```python
from build123d import *

# Parameters (mm, degrees)
SKETCH1_W           = 12.710924787
SKETCH1_H           = 15.963552005
SKETCH1_R           = 1.8
BOSS_EXTRUDE1_DEPTH = 1
SKETCH2_R           = 1.75
BOSS_EXTRUDE2_DEPTH = 5
SKETCH3_R           = 3.5
BOSS_EXTRUDE3_DEPTH = 5
CHAMFER1_SIZE       = 2


with BuildPart() as part:
    # Sketch1 → Boss-Extrude1 (new body)
    with BuildSketch(Plane.XY.offset(46.41148)):
        with Locations((39.508303211, 7.326783953)):
            Rectangle(SKETCH1_W, SKETCH1_H)
        with Locations((38.478852397, 6.566573863)):
            Circle(SKETCH1_R, mode=Mode.SUBTRACT)
    extrude(amount=BOSS_EXTRUDE1_DEPTH)

    # Sketch2 → Boss-Extrude2 (add)
    with BuildSketch(Plane(origin=(30.5, 0, 0), x_dir=(0, 0, -1), z_dir=(1, 0, 0))):
        with BuildLine():
            Line((-56.841529107, 37.437587441), (-49.41148, 37.437587441))
            Line((-49.41148, 37.437587441), (-49.41148, 17.308559955))
            Line((-49.41148, 17.308559955), (-47.41148, 15.308559955))
            Line((-47.41148, 15.308559955), (-47.41148, 12.308559955))
            Line((-47.41148, 12.308559955), (-52.41148, 12.308559955))
            Line((-52.41148, 12.308559955), (-61.318087937, 30.210387171))
            ThreePointArc((-61.318087937, 30.210387171), (-61.092176196, 35.07045647), (-56.841529107, 37.437587441))
        make_face()
        with Locations((-56.841529107, 32.437587441)):
            Circle(SKETCH2_R, mode=Mode.SUBTRACT)
    extrude(amount=BOSS_EXTRUDE2_DEPTH)

    # Sketch3 → Boss-Extrude3 (add)
    with BuildSketch(Plane.XY.offset(47.41148)):
        Polygon((35.5, 15.308559955), (35.5, 12.308559955), (33.152840817, 12.308559955), (33.152840817, -0.65499205), (45.863765604, -0.65499205), (45.863765604, 15.308559955), align=None)
        with Locations((38.478852397, 6.566573863)):
            Circle(SKETCH3_R, mode=Mode.SUBTRACT)
    extrude(amount=BOSS_EXTRUDE3_DEPTH)

    # Chamfer1
    chamfer1_edges = [part.edges().sort_by_distance(p)[0] for p in [
        (33.152840817, 12.308559955, 49.91148),
    ]]
    chamfer(chamfer1_edges, length=CHAMFER1_SIZE)


solid = part.part
```
Geometry check sheet. Reference: the model listing, model coordinates, mm. A direction names the side the tool comes from. Coordinates: 2 decimals unless noted, no trailing zeros. Order: outer loops, then holes, each group sorted by start corner. A loop starts at its lowest first (then second) coordinate and runs counter-clockwise, first axis right, second up.
Q1. Sectioned sample at A-A on z = 57.5. Record the cut outline in (x, y).
Reply:
outline: (30.5, 22.54) - (35.5, 22.54) - (35.5, 30.82) - (30.5, 30.82) - close; (30.5, 34.06) - (35.5, 34.06) - (35.5, 37.39) - (30.5, 37.39) - close
Q2. Thickness scan on probe 1 along X at (y, z) = (26, 51.5); probe 2 along Z at (x, y) = (42.5, 7); probe 3 along Y at (x, z) = (33, 56.75). Record the ranges inside material, lowest first.
Reply:
probe 1: x = 30.5 to 35.5
probe 2: z = 46.41 to 52.41
probe 3: y = 21.03 to 30.69, 34.19 to 37.44
Q3. Draft check along Y on faces 1 (the face through (33.153, 5, 49)), 2 (the face through (40.2, 7.1, 46.9)), 3 (the face through (32.965, 33.913, 55.901)), 4 (the face through (41, 15.309, 49)). Enter one of: released by +Y, released by -Y, zero draft, split by the parting line, or undercut.
Reply:
face 1: zero draft
face 2: undercut
face 3: undercut
face 4: released by +Y
Q4. Sectioned sample at C-C on z = 49. Record the cut outline in (x, y) (3 decimals), and give its area (3 significant figures).
Reply:
outline: (30.5, 12.309) - (31.153, 12.309) - (33.153, 10.309) - (33.153, -0.655) - (45.864, -0.655) - (45.864, 15.309) - (35.5, 15.309) - (35.5, 16.897) - (30.5, 16.897) - close; hole circle Ø7 at (38.479, 6.567)
area: 182 mm2
Q5. Depth check by flat-ended pin: pin 1 Ø5 at (x, y) = (43, 5) entering from +Z; pin 2 Ø3 at (x, z) = (36.5, 48) entering from +Y; pin 3 Ø1.3 at (x, y) = (32, 12) entering from -Z. Enter the tip coordinate at first touch or a pass-through.
Reply:
pin 1: stops at z = 52.41
pin 2: stops at y = 17.02
pin 3: stops at z = 47.41
Q6. Sectioned sample at B-B on y = 8. Record the cut outline in (x, z), and give its area (3 significant figures).
Reply:
outline: (33.15, 46.41) - (37.39, 46.41) - (37.39, 47.41) - (35.29, 47.41) - (35.29, 52.41) - (33.15, 52.41) - close; (39.57, 46.41) - (45.86, 46.41) - (45.86, 52.41) - (41.67, 52.41) - (41.67, 47.41) - (39.57, 47.41) - close
area: 42.2 mm2
Q7. Tool access check on faces 5 (the face through (32, 13, 47.411)), 6 (the face through (42, 9, 52.411)), 7 (the face through (41.817, 7.618, 49.876)). Record the directions out of +Z, -Z, +X, -X, +Y, -Y that give a thin tool (end or side, any length) a straight path to the whole face; none if there is none.
Reply:
face 5: -Z, -X, +Y, -Y
face 6: +Z, +X, -Y
face 7: +Z
Q8. Sectioned sample at D-D on x = 36. Record the cut outline in (y, z) (3 decimals).
Reply:
outline: (-0.655, 46.411) - (15.309, 46.411) - (15.309, 52.411) - (9.037, 52.411) - (9.037, 47.411) - (4.096, 47.411) - (4.096, 52.411) - (-0.655, 52.411) - close
